Check sheet for the modelled part. Datum: model origin and axes. Units: mm. A direction names the side the tool comes from. Round coordinates to 2 decimals unless told otherwise and drop trailing zeros. Write each loop counter-clockwise with the first axis right and the second up, starting at its lowest first coordinate (ties: lowest second). Pieces come first, ordered by that corner, then holes. Notation, with made-up numbers: (-36, 83) -> (23, 83) arc R27 ccw to (23, 101) -> close; hole circle Ø2 at (10.25, 28). An arc over 180 degrees is marked (long way). Answer as a JSON object with one key per item and string values. Group by question number.
```python
from build123d import *

# Parameters (mm, degrees)
SKETCH1_R           = 2
SKETCH1_R_2         = 1.143
SKETCH1_W           = 12.7
SKETCH1_H           = 50.8
BOSS_EXTRUDE3_DEPTH = 6.35


with BuildPart() as part:
    # Sketch1 → Boss-Extrude3 (new body)
    with BuildSketch(Plane(origin=(0, 0, 0), x_dir=(1, 0, 0), z_dir=(0, 1, 0))):
        with BuildLine():
            ThreePointArc((32.240681933, -66.10056535), (0, -48.302004425), (-32.240681933, -66.10056535))
            ThreePointArc((-32.240681933, -66.10056535), (-33.11372382, -66.748004461), (-34.194833578, -66.63583839))
            ThreePointArc((-34.194833578, -66.63583839), (0, 74.897407173), (34.194833578, -66.63583839))
            ThreePointArc((34.194833578, -66.63583839), (33.11372382, -66.748004461), (32.240681933, -66.10056535))
        make_face()
        with Locations((-18.178952795, 24.310551096)):
            Circle(SKETCH1_R, mode=Mode.SUBTRACT)
        with Locations((-46.663733983, -40.081231883)):
            Circle(SKETCH1_R, mode=Mode.SUBTRACT)
        with Locations((46.663733983, -40.081231883)):
            Circle(SKETCH1_R, mode=Mode.SUBTRACT)
        with Locations((46.663733983, 40.081231883)):
            Circle(SKETCH1_R, mode=Mode.SUBTRACT)
        with Locations((-46.663733983, 40.081231883)):
            Circle(SKETCH1_R, mode=Mode.SUBTRACT)
        with Locations((-6.731, 64.107698843)):
            Circle(SKETCH1_R_2, mode=Mode.SUBTRACT)
        with Locations((6.731, 64.107698843)):
            Circle(SKETCH1_R_2, mode=Mode.SUBTRACT)
        with Locations((18.178952795, 24.310551096)):
            Circle(SKETCH1_R, mode=Mode.SUBTRACT)
        with Locations((0, 53.061187965)):
            Circle(SKETCH1_R, mode=Mode.SUBTRACT)
        with Locations((61.164123727, 0)):
            Rectangle(SKETCH1_W, SKETCH1_H, mode=Mode.SUBTRACT)
        with Locations((-61.164123727, 0)):
            Rectangle(SKETCH1_W, SKETCH1_H, mode=Mode.SUBTRACT)
    extrude(amount=BOSS_EXTRUDE3_DEPTH)


solid = part.part
```
(1) Section check B-B on z = 0. Record the cut outline in (x, y), then the cut area to 3 significant figures.
(2) Go/stop test with flat-tipped pins: pin 1 Ø2.5 at (x, z) = (-46.66, -40.08) entering from -Y; pin 2 Ø1.5 at (y, z) = (5, 41.5) entering from +X; pin 3 Ø3 at (y, z) = (5.5, 18.5) entering from -X; pin 4 Ø1.9 at (y, z) = (3.5, 5) entering from -X. Record where each tip stops, or that it passes through.
(3) Section check C-C on y = 2.5. State how many separate pieces and enclosed holes the cut face has, then the cut area to 3 significant figures.
(4) Scan lines: line 1 along X through (y, z) = (6.25, 2); line 2 along X through (y, z) = (5.25, 15); line 3 along Z through (x, y) = (55, 5.75). Record each from-to range of solid material in increasing order.
(5) Section check A-A on x = 0. Record the cut outline in (y, z).
(6) Access from +Z, -Z, +X, -X, +Y, -Y to the whole of each face (thin tool, end or side, straight path). Record for faces 1 (the cylindrical face through (0.538, 3.131, 48.306)), 2 (the flat face through (61, 3, -25.4)).
(7) Release check for a two-part mould opening along X. For faces 3 (the cylindrical face through (-2.796, 3.131, -74.845)), 4 (the cylindrical face through (0.923, 3.131, -51.287)), 5 (the flat face through (1, 0, -5)) record: pulls with the +X half, pulls with the -X half, needs draft (parallel to the pull), parting line crosses it, or undercut.
(8) Section check D-D on x = -57.5. Record the cut outline in (y, z).
Data:
{
 "1": {"outline": "(-74.9, 0) -> (-67.51, 0) -> (-67.51, 6.35) -> (-74.9, 6.35) -> close; (-54.81, 0) -> (54.81, 0) -> (54.81, 6.35) -> (-54.81, 6.35) -> close; (67.51, 0) -> (74.9, 0) -> (74.9, 6.35) -> (67.51, 6.35) -> close", "area": "790 mm²"},
 "2": {"pin 1": "passes through", "pin 2": "stops at x = 62.84", "pin 3": "stops at x = -72.94", "pin 4": "stops at x = -74.79"},
 "3": {"separate pieces": "1", "enclosed holes": "11", "area": "15,000 mm²"},
 "4": {"line 1": "x = -74.87 to -67.51, -54.81 to 54.81, 67.51 to 74.87", "line 2": "x = -73.38 to -67.51, -54.81 to 54.81, 67.51 to 73.38", "line 3": "z = -50.84 to -25.4, 25.4 to 50.84"},
 "5": {"outline": "(0, -74.9) -> (6.35, -74.9) -> (6.35, -55.06) -> (0, -55.06) -> close; (0, -51.06) -> (6.35, -51.06) -> (6.35, 48.3) -> (0, 48.3) -> close"},
 "6": {"face 1": "+Z, +Y, -Y", "face 2": "+Y, -Y"},
 "7": {"face 3": "parting line crosses it", "face 4": "undercut", "face 5": "needs draft"},
 "8": {"outline": "(0, -47.99) -> (6.35, -47.99) -> (6.35, -25.4) -> (0, -25.4) -> close; (0, 25.4) -> (6.35, 25.4) -> (6.35, 47.99) -> (0, 47.99) -> close"}
}
